Job drawing, mm, ordinate dimensions from the low corner. One solid piece. Coordinates: 2 decimals unless noted, no trailing zeros. Loops run counter-clockwise (first coordinate to the right, second up) from the corner with the lowest first, then second, coordinate; pieces in that order, holes last. Notation, with made-up numbers: (59.25, 54.5) - (78.25, 54.5) arc R21 cw to (78.25, 79.5) - close; hole circle Ø6 at (10, 11). An arc over 180 degrees is marked (long way). Use a Markdown table: item, result. Add a question column.
1. Wall check: probe 1 along X at (y, z) = (6.5, 3); probe 2 along X at (y, z) = (17, 19.75) (1 decimal); probe 3 along Y at (x, z) = (4.5, 10.5) (1 decimal). Give the ranges that are in metal, low to high. Write a range as [from, to].
2. Band-saw the part on A-A, the plane z = 6.25. Give the cut face in (x, y).
3. Band-saw the part on B-B, the plane y = 10.5. Give the cut face in (x, z).
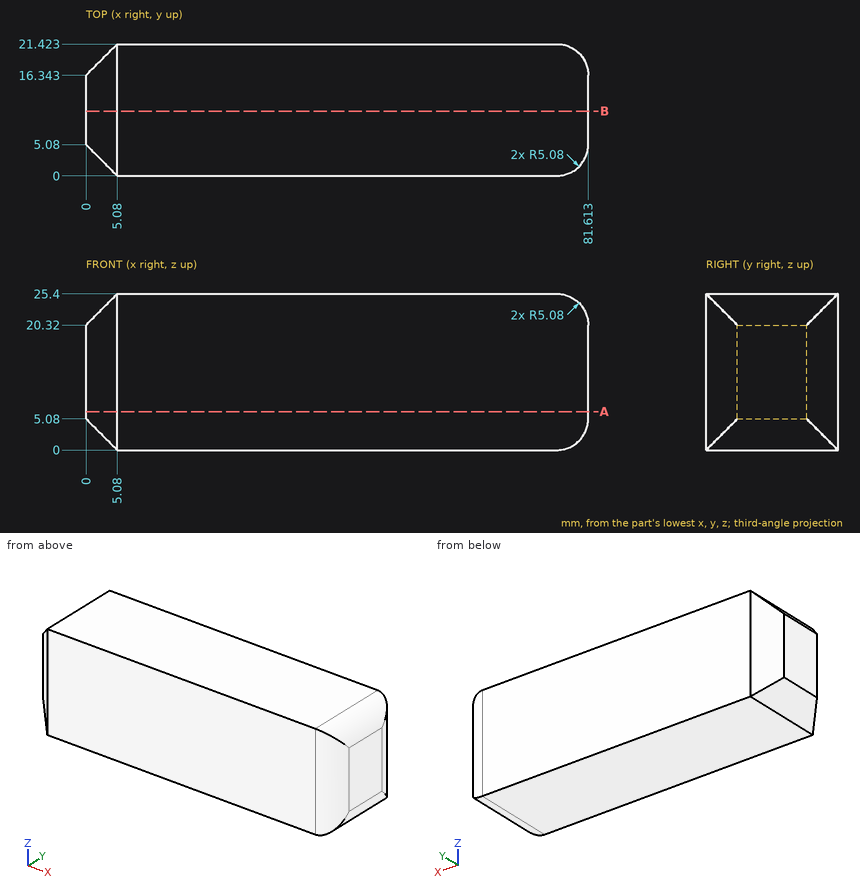
Geometry check:
| question | item | result |
|---|---|---|
| 1 | probe 1 | x = [2.08, 81.17] |
| 1 | probe 2 | x = [0.7, 81.6] |
| 1 | probe 3 | y = [0.6, 20.8] |
| 2 | outline | (0, 5.08) - (5.08, 0) - (76.53, 0) arc R5.08 ccw to (81.61, 5.08) - (81.61, 16.34) arc R5.08 ccw to (76.53, 21.42) - (5.08, 21.42) - (0, 16.34) - close |
| 3 | outline | (0, 5.08) - (5.08, 0) - (76.53, 0) arc R5.08 ccw to (81.61, 5.08) - (81.61, 20.32) arc R5.08 ccw to (76.53, 25.4) - (5.08, 25.4) - (0, 20.32) - close |
